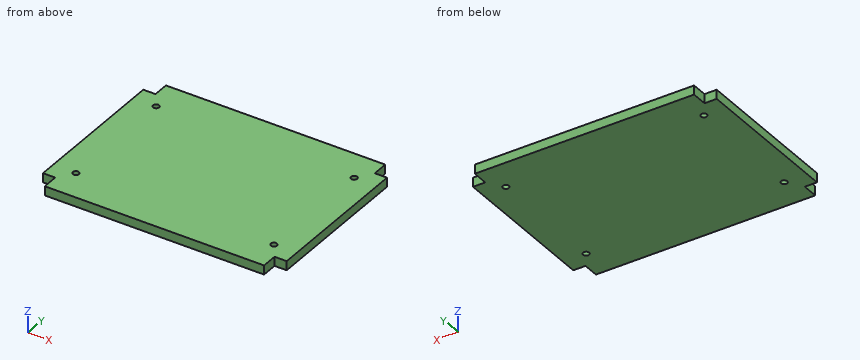
Autodesk Inventor part; units mm, degrees
ref_plane "YZ Plane" through (0, 0, 0) normal (1, 0, 0) x (0, 1, 0)
ref_plane "XZ Plane" through (0, 0, 0) normal (0, 1, 0) x (-1, 0, 0)
ref_plane "XY Plane" through (0, 0, 0) normal (0, 0, 1) x (1, 0, 0)
sketch "Skizze1" plane through (0, 0, 0) normal (0, 0, 1) x (1, 0, 0)
  line L0 (-102.3641, 100) -> (-101.6, 100) construction
  line L1 (-101.6, 0) -> (-102.3641, 0) construction
  line L2 (19.2, -16.0826) -> (-120.8, -16.0826) construction
  line L3 (-120.8, -16.0826) -> (-120.8, -13.8079) construction
  line L4 (-120.8, -13.8079) -> (19.2, -13.8079) construction
  line L5 (19.2, -13.8079) -> (19.2, -16.0826) construction
  line L6 (19.2, -28.3315) -> (-120.8, -28.3315) construction
  line L7 (-120.8, -28.3315) -> (-120.8, -24.6314) construction
  line L8 (-120.8, -24.6314) -> (19.2, -24.6314) construction
  line L9 (19.2, -24.6314) -> (19.2, -28.3315) construction
  line L10 (-120.8, 124.6314) -> (-120.8, 128.3315) construction
  line L11 (19.2, 128.3315) -> (19.2, 124.6314) construction
  line L12 (19.2, 116.0826) -> (19.2, 113.8079) construction
  line L13 (0, 100) -> (0.7641, 100) construction
  line L14 (0.7641, 0) -> (0, 0) construction
  line L15 (17.6359, 100) -> (18.4, 100) construction
  line L16 (18.4, 0) -> (17.6359, 0) construction
  line L17 (5.1816, 100) -> (13.2184, 100) construction
  line L18 (13.2184, 0) -> (5.1816, 0) construction
  line L19 (69.2, -3.3397) -> (-120.8, -3.3397) construction
  line L20 (69.2, 103.3397) -> (-120.8, 103.3397) construction
  line L21 (-105.8, 0.0011) -> (54.2, 0.0011)
  line L22 (54.2, 0.0011) -> (54.2, 100.0011)
  line L23 (54.2, 100.0011) -> (-105.8, 100.0011)
  line L24 (-105.8, 100.0011) -> (-105.8, 0.0011)
  line L25 (69.2, -9.3201) -> (-120.8, -9.3201) construction
  line L26 (69.2, 109.0272) -> (-120.8, 109.0272) construction
  line L27 (-100.8, -12.3397) -> (-100.8, 0) construction
  line L28 (49.2, 0) -> (49.2, -12.3397) construction
  line L29 (-100.8, -10.3935) -> (49.2, -10.3935)
  line L30 (49.2, -10.3935) -> (49.2, 110.3935)
  line L31 (49.2, 110.3935) -> (-100.8, 110.3935)
  line L32 (-100.8, 110.3935) -> (-100.8, -10.3935)
  line L33 (-120.8, -7.2256) -> (69.2, -7.2256)
  line L34 (74.2, 45.0011) -> (74.2, -28.46)
  line L35 (74.2, -28.46) -> (69.2, -28.46)
  line L36 (69.2, -28.46) -> (69.2, -6.9656)
  line L37 (69.2, -6.9656) -> (49.2, -6.9656)
  line L38 (49.2, -6.9656) -> (49.2, 0.0011)
  line L39 (49.2, 0.0011) -> (69.2, 0.0011)
  line L40 (69.2, 0.0011) -> (69.2, 45.0011)
  line L41 (69.2, 45.0011) -> (74.2, 45.0011)
  line L42 (69.2, 110.3935) -> (-120.8, 110.3935)
  line L43 (69.2, -11.4055) -> (69.2, -10.3935)
  line L44 (69.2, -10.3935) -> (-120.8, -10.3935)
  dimension "d2" = 5
  dimension "d3" = 5
  dimension "d4" = 100
extrude "Extrusion1" add sketch "Skizze1" along normal blind 6 contours L30 L23 L22 L21 | L30 L33 L32 L21 | L21 L32 L23 L30 | L21 L24 L23 L32 | L23 L32 L31 L30 | L33 L30 L29 L32
sketch "Skizze2" plane through (0, 0, 6) normal (0, 0, 1) x (1, 0, 0)
  line L0 (49.2, 100.0011) -> (49.2, 110.3935)
  line L1 (-100.8, 110.3935) -> (-100.8, 100.0011)
  line L2 (-100.8, 100.0011) -> (-105.8, 100.0011)
  line L3 (-105.8, 0.0011) -> (-100.8, 0.0011)
  line L4 (-100.8, 0.0011) -> (-100.8, -10.3935)
  line L5 (49.2, -10.3935) -> (49.2, 0.0011)
  line L6 (49.2, 0.0011) -> (54.2, 0.0011)
  line L7 (54.2, 100.0011) -> (49.2, 100.0011)
  point P0 (0, 0)
  point P1 (39.2, 10.0011)
  point P2 (39.2, 90.0011)
  point P3 (-90.8, 90.0011)
  point P4 (-90.8, 10.0011)
  dimension "d5" = 10
  dimension "d6" = 10
  dimension "d7" = 10
  dimension "d8" = 10
  dimension "d9" = 10
  dimension "d10" = 10
  dimension "d11" = 10
  dimension "d12" = 10
hole "Bohrung1" at (39.2, 10.0011, 6) at (39.2, 90.0011, 6) at (-90.8, 90.0011, 6) at (-90.8, 10.0011, 6) direction (0, 0, -1) diameter 4 end through all
sketch "Skizze3" plane through (0, 0, 0) normal (0, 0, -1) x (-1, 0, 0)
  line L0 (105.8, 0.0011) -> (100.8, 0.0011)
  line L1 (100.8, 110.3935) -> (100.8, 100.0011)
  line L2 (-49.2, 110.3935) -> (100.8, 110.3935)
  line L3 (-49.2, 100.0011) -> (-49.2, 110.3935)
  line L4 (-49.2, -10.3935) -> (-49.2, 0.0011)
  line L5 (100.8, -10.3935) -> (-49.2, -10.3935)
  line L6 (100.8, 0.0011) -> (100.8, -10.3935)
  line L7 (-49.2, 100.0011) -> (-46.2, 100.0011)
  line L8 (-46.2, 100.0011) -> (-46.2, 110.3935)
  line L9 (-49.2, 0.0011) -> (-46.2, 0.0011)
  line L10 (-46.2, 0.0011) -> (-46.2, -10.3935)
  line L11 (97.8, -10.3935) -> (97.8, 0.0011)
  line L12 (97.8, 0.0011) -> (100.8, 0.0011)
  line L13 (100.8, 100.0011) -> (97.8, 100.0011)
  line L14 (97.8, 100.0011) -> (97.8, 110.3935)
  point P0 (0, 0)
  dimension "d20" = 3
  dimension "d21" = 3
extrude "Extrusion2" cut sketch "Skizze3" against normal through all
equation "\"d2\" = d3"
equation "\"d21\" = d20"
properties part number "SeitenWand" material "Holz (Birke)"
Build history of the part. All positions in model axes, mm. Coordinates: 2 decimals unless noted, no trailing zeros. Order: outer loops, then holes, each group sorted by start corner. A loop starts at its lowest first (then second) coordinate and runs counter-clockwise, first axis right, second up. Notation, with made-up numbers: (8, 31) -> (66, 31) arc R30 cw to (66, 70) -> close; hole circle Ø11 at (10, 68.25). An arc over 180 degrees is marked (long way). Answer in a Markdown table with one row per item. Add a question column.
Q1. Band-saw the part on B-B, the plane z = 3.4. List the corners of the cut face in (x, y), then the cut area to 3 significant figures.
Q2. Band-saw the part on A-A, the plane x = 39.2. List the corners of the cut face in (y, z).
Q3. Wall check: line 1 along Y through (x, z) = (39.2, 3.6); line 2 along X through (y, z) = (-2.5, 4.5). Give the ranges that are in metal, low to high. Write a range as [from, to].
Q4. Drop flat-ended pins along their axis: pin 1 (3 mm diameter, centred on y = 105.5, z = 2.5, fed in from +X); pin 2 (3 mm diameter, centred on x = 39.2, y = 10, fed in from -Z). Give the stop position or say it passes through.
Answers follow:
| question | item | result |
|---|---|---|
| 1 | outline | (-105.8, 0) -> (-97.8, 0) -> (-97.8, -10.39) -> (46.2, -10.39) -> (46.2, 0) -> (54.2, 0) -> (54.2, 100) -> (46.2, 100) -> (46.2, 110.39) -> (-97.8, 110.39) -> (-97.8, 100) -> (-105.8, 100) -> close; hole circle Ø4 at (-90.8, 10); hole circle Ø4 at (-90.8, 90); hole circle Ø4 at (39.2, 10); hole circle Ø4 at (39.2, 90) |
| 1 | area | 18,900 mm^2 |
| 2 | outline | (-10.39, 0) -> (8, 0) -> (8, 6) -> (-10.39, 6) -> close; (12, 0) -> (88, 0) -> (88, 6) -> (12, 6) -> close; (92, 0) -> (110.39, 0) -> (110.39, 6) -> (92, 6) -> close |
| 3 | line 1 | [-10.39, 8], [12, 88], [92, 110.39] |
| 3 | line 2 | [-97.8, 46.2] |
| 4 | pin 1 | x = 46.2 |
| 4 | pin 2 | through |
